Here's the drawing with two shaded views (mm, measured from the low corner). I have some questions. Round coordinates to 2 decimals unless told otherwise and drop trailing zeros. Order: outer loops, then holes, each group sorted by start corner. A loop starts at its lowest first (then second) coordinate and runs counter-clockwise, first axis right, second up. Notation, with made-up numbers: (3, 80.25) -> (19, 80.25) arc R28 ccw to (19, 101.25) -> close; hole circle Ø1 at (11, 50.25). An arc over 180 degrees is marked (long way). Answer in a Markdown table with one row per item.
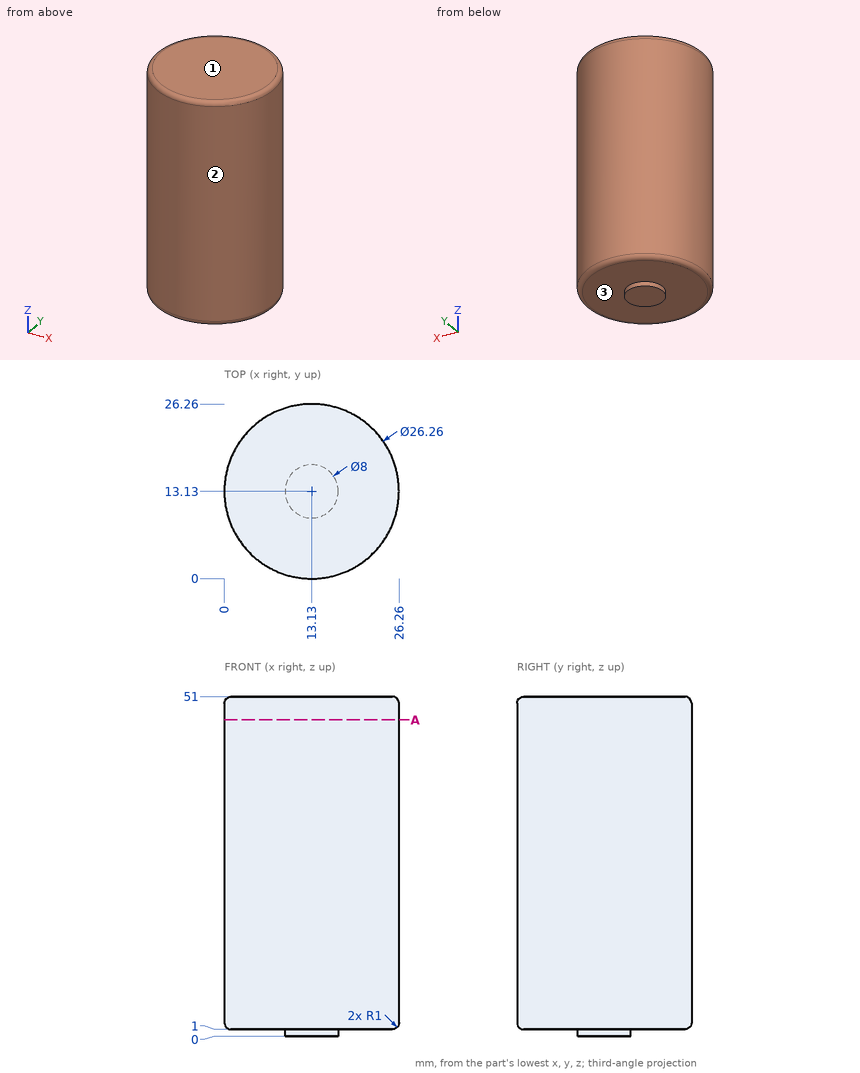
1. Suppose I cut it at A-A on z = 47.5. Write out the boundary of the cut face in (x, y), then the cut area to 3 significant figures.
Numbers:
| item | result |
|---|---|
| outline | circle Ø26.26 at (13.13, 13.13) |
| area | 542 mm2 |
2. Please list where these lines run through material, in increasing order: line 1 along Z through (x, y) = (4.5, 21.75); line 2 along Y through (x, z) = (13, 44.5); line 3 along X through (y, z) = (21.25, 11.5).
Numbers:
| item | result |
|---|---|
| line 1 | z = 1 to 51 |
| line 2 | y = 0 to 26.26 |
| line 3 | x = 2.81 to 23.45 |
3. We'd pull the mould along Z, two halves only. Please class the marked faces 1, 2 and 3: released by +Z, released by -Z, zero draft, split by the parting line, or undercut.
Numbers:
| item | result |
|---|---|
| face 1 | released by +Z |
| face 2 | zero draft |
| face 3 | released by -Z |
4. For pin 1 Ø1.5 at (y, z) = (11, 32) entering from +X; pin 2 Ø12 at (x, z) = (23.5, 33) entering from -Y; pin 3 Ø12 at (x, z) = (22.5, 22.5) entering from -Y, each with a flat end and sliding along its axis, tell me the tip position at first contact or that it passes through.
Numbers:
| item | result |
|---|---|
| pin 1 | stops at x = 26.19 |
| pin 2 | stops at y = 0.75 |
| pin 3 | stops at y = 0.44 |
